```python
from build123d import *

# Parameters (mm, degrees)
SKETCH_W        = 93
SKETCH_H        = 130
SKETCH_R        = 1.5
SKETCH_R_2      = 2
PAD_DEPTH       = 3
SKETCH001_W     = 3
SKETCH001_H     = 130
PAD001_DEPTH    = 30
SKETCH002_R     = 3
POCKET_DEPTH    = 3.001
CHAMFER_SIZE    = 2
CHAMFER001_SIZE = 4


with BuildPart() as part:
    # Sketch → Pad (new body)
    with BuildSketch(Plane.XY):
        with Locations((46.5, 65)):
            Rectangle(SKETCH_W, SKETCH_H)
        with Locations((20.5, 30)):
            Circle(SKETCH_R, mode=Mode.SUBTRACT)
        with Locations((68, 110)):
            Circle(SKETCH_R, mode=Mode.SUBTRACT)
        with Locations((8, 125)):
            Circle(SKETCH_R_2, mode=Mode.SUBTRACT)
        with Locations((88, 125)):
            Circle(SKETCH_R_2, mode=Mode.SUBTRACT)
        with Locations((88, 5)):
            Circle(SKETCH_R_2, mode=Mode.SUBTRACT)
        with Locations((8, 5)):
            Circle(SKETCH_R_2, mode=Mode.SUBTRACT)
    extrude(amount=PAD_DEPTH)

    # Sketch001 (on Face12 of Pad) → Pad001 (join)
    with BuildSketch(Plane.XY.offset(3)):
        with Locations((1.5, 65)):
            Rectangle(SKETCH001_W, SKETCH001_H)
    extrude(amount=PAD001_DEPTH)

    # Sketch002 (on Face15 of Pad001) → Pocket (cut, through all)
    with BuildSketch(Plane.YZ.offset(3)):
        with Locations((30, 18)):
            Circle(SKETCH002_R)
        with Locations((100, 18)):
            Circle(SKETCH002_R)
    extrude(amount=-POCKET_DEPTH, mode=Mode.SUBTRACT)

    # Chamfer
    chamfer_edges = [part.edges().sort_by_distance(p)[0] for p in [
        (93, 0, 1.5),
        (93, 130, 1.5),
    ]]
    chamfer(chamfer_edges, length=CHAMFER_SIZE)

    # Chamfer001
    chamfer001_edges = [part.edges().sort_by_distance(p)[0] for p in [
        (1.5, 0, 33),
        (1.5, 130, 33),
    ]]
    chamfer(chamfer001_edges, length=CHAMFER001_SIZE)


solid = part.part
```
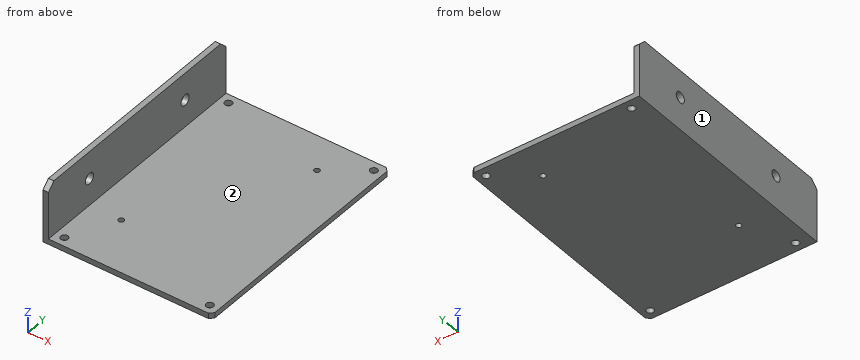
Check sheet for the modelled part. Datum: model origin and axes. Units: mm. Face numbers are marked on the shaded views. A direction names the side the tool comes from. Give positions to 0.01 mm unless a question says otherwise; leave off trailing zeros. Write each loop counter-clockwise with the first axis right and the second up, starting at its lowest first coordinate (ties: lowest second). Pieces come first, ordered by that corner, then holes.
Item 1: Cross-section at C-C (x = 88). Enter the section's corners in (y, z).
Item 2: Gauge pin test, flat ends, axial feed: pin 1 (6 mm diameter, centred on y = 86, z = 17.5, fed in from +X); pin 2 (3 mm diameter, centred on x = 88, y = 125, fed in from +Z); pin 3 (3.5 mm diameter, centred on x = 68, y = 110, fed in from +Z). Record the tip position at first contact, or that the pin passes through.
Item 3: Cross-section at A-A (z = 18). Enter the section's corners in (x, y).
Item 4: Scan lines: L1, parallel to Y at x = 8, z = 0.9; L2, parallel to Z at x = 1, y = 30; L3, parallel to Z at x = 19, y = 77.5. Record each from-to range of solid material in increasing order.
Item 5: Cross-section at B-B (y = 30). Enter the section's corners in (x, z), and give its area (3 significant figures).
Item 6: Access from +Z, -Z, +X, -X, +Y, -Y to the whole of each face (thin tool, end or side, straight path). Record for the marked faces 1 and 2.
Item 7: Cross-section at D-D (y = 100). Enter the section's corners in (x, z).
Report:
1. outline: (0, 0) - (3, 0) - (3, 3) - (0, 3) - close; (7, 0) - (123, 0) - (123, 3) - (7, 3) - close; (127, 0) - (130, 0) - (130, 3) - (127, 3) - close
2. pin 1: stops at x = 3
2. pin 2: passes through
2. pin 3: stops at z = 3
3. outline: (0, 0) - (3, 0) - (3, 27) - (0, 27) - close; (0, 33) - (3, 33) - (3, 97) - (0, 97) - close; (0, 103) - (3, 103) - (3, 130) - (0, 130) - close
4. L1: y = 0 to 3, 7 to 123, 127 to 130
4. L2: z = 0 to 15, 21 to 33
4. L3: z = 0 to 3
5. outline: (0, 0) - (19, 0) - (19, 3) - (3, 3) - (3, 15) - (0, 15) - close; (0, 21) - (3, 21) - (3, 33) - (0, 33) - close; (22, 0) - (93, 0) - (93, 3) - (22, 3) - close
5. area: 342 mm2
6. face 1: +Z, -Z, -X, +Y, -Y
6. face 2: +Z, +X, +Y, -Y
7. outline: (0, 0) - (93, 0) - (93, 3) - (3, 3) - (3, 15) - (0, 15) - close; (0, 21) - (3, 21) - (3, 33) - (0, 33) - close
